Read the model definition and answer for the solid it produces. Units are mm, in the model's axes. A direction names the side the tool comes from. Give positions to 0.01 mm unless a question says otherwise; leave off trailing zeros. Loops run counter-clockwise (first coordinate to the right, second up) from the corner with the lowest first, then second, coordinate; pieces in that order, holes last. Notation, with made-up numbers: (14.5, 21.5) - (27.5, 21.5) arc R9 cw to (27.5, 26.5) - close; hole circle Ø10 at (68, 42). An arc over 180 degrees is marked (long way). Write item = value, one per line.
Autodesk Inventor part; units mm, degrees
ref_plane "YZ Plane" through (0, 0, 0) normal (1, 0, 0) x (0, 1, 0)
ref_plane "XZ Plane" through (0, 0, 0) normal (0, 1, 0) x (-1, 0, 0)
ref_plane "XY Plane" through (0, 0, 0) normal (0, 0, 1) x (1, 0, 0)
sketch "스케치1" plane through (0, 0, 0) normal (0, 0, 1) x (1, 0, 0)
  line L0 (-8.75, -14) -> (8.75, -14)
  line L1 (8.75, -14) -> (8.75, 14)
  line L2 (8.75, 14) -> (-8.75, 14)
  line L3 (-8.75, 14) -> (-8.75, -14)
  line L4 (-8.75, -14) -> (8.75, 14) construction
  line L5 (8.75, -14) -> (-8.75, 14) construction
  line L6 (-8.75, -14) -> (-6.31, -14)
  line L7 (-6.31, -14) -> (-6.31, -12.46)
  line L8 (-6.31, -12.46) -> (0, -12.46)
  line L9 (0, 0) -> (0, 2.6603)
  line L10 (8.75, -14) -> (6.31, -14)
  line L11 (6.31, -14) -> (6.31, -12.46)
  line L12 (6.31, -12.46) -> (0, -12.46)
  dimension "d0" = 17.5
  dimension "d1" = 28
  dimension "d2" = 2.44
  dimension "d3" = 1.54
extrude "돌출1" add sketch "스케치1" along normal blind 1 contours L3 L2 L1 L0 L11 L12 L8 L7
sketch "스케치2" plane through (-8.75, 14, 0) normal (0, 1, 0) x (1, 0, 0)
  line L0 (5.2, -1) -> (12.3, -1)
  line L1 (13.3, -2) -> (13.3, -3.15)
  line L2 (12.3, -4.15) -> (5.2, -4.15)
  line L3 (4.2, -3.15) -> (4.2, -2)
  line L4 (4.2, -1) -> (13.3, -4.15) construction
  line L5 (13.3, -1) -> (4.2, -4.15) construction
  line L6 (17.5, -1) -> (0, -1) construction
  line L7 (6.25, -2.075) -> (11.25, -2.075)
  line L8 (11.25, -2.075) -> (11.25, -3.075)
  line L9 (11.25, -3.075) -> (6.25, -3.075)
  line L10 (6.25, -3.075) -> (6.25, -2.075)
  line L11 (6.25, -2.075) -> (11.25, -3.075) construction
  line L12 (11.25, -2.075) -> (6.25, -3.075) construction
  arc A0 (13.3, -2) -> (12.3, -1) centre (12.3, -2) ccw
  arc A1 (12.3, -4.15) -> (13.3, -3.15) centre (12.3, -3.15) ccw
  arc A2 (5.2, -1) -> (4.2, -2) centre (5.2, -2) ccw
  arc A3 (4.2, -3.15) -> (5.2, -4.15) centre (5.2, -3.15) ccw
  line L13 (13.1, -3.15) -> (13.1, -2)
  arc A4 (13.1, -2) -> (12.3, -1.2) centre (12.3, -2) ccw
  line L14 (12.3, -1.2) -> (5.2, -1.2)
  arc A5 (5.2, -1.2) -> (4.4, -2) centre (5.2, -2) ccw
  line L15 (4.4, -2) -> (4.4, -3.15)
  arc A6 (4.4, -3.15) -> (5.2, -3.95) centre (5.2, -3.15) ccw
  line L16 (5.2, -3.95) -> (12.3, -3.95)
  arc A7 (12.3, -3.95) -> (13.1, -3.15) centre (12.3, -3.15) ccw
  point P0 (8.75, 0)
  point P1 (8.75, -2.575)
  point P2 (8.75, -1)
  dimension "d6" = 3.15
  dimension "d7" = 9.1
  dimension "d8" = 5
  dimension "d9" = 1
  dimension "d10" = 1
  dimension "d11" = 0.2
extrude "돌출2" add sketch "스케치2" along normal blind 1.74 and the other way blind 5.86
fillet "모깎기1" radius 0.7 2 edges at (6.31, -12.46, 0.5) (-6.31, -12.46, 0.5)
sketch "스케치3" plane through (-8.75, 8.14, 0) normal (0, -1, 0) x (1, 0, 0)
  line L0 (12.3, 4.15) -> (5.2, 4.15)
  arc A0 (5.2, 4.15) -> (4.2, 3.15) centre (5.2, 3.15) ccw
  line L1 (4.2, 3.15) -> (4.2, 2)
  arc A1 (4.2, 2) -> (5.2, 1) centre (5.2, 2) ccw
  line L2 (12.3, 1) -> (5.2, 1)
  arc A2 (12.3, 1) -> (13.3, 2) centre (12.3, 2) ccw
  line L3 (13.3, 2) -> (13.3, 3.15)
  arc A3 (13.3, 3.15) -> (12.3, 4.15) centre (12.3, 3.15) ccw
  arc A4 (13.1, 3.15) -> (12.3, 3.95) centre (12.3, 3.15) ccw
  line L4 (13.1, 3.15) -> (13.1, 2)
  arc A5 (12.3, 1.2) -> (13.1, 2) centre (12.3, 2) ccw
  line L5 (12.3, 1.2) -> (5.2, 1.2)
  arc A6 (4.4, 2) -> (5.2, 1.2) centre (5.2, 2) ccw
  line L6 (4.4, 2) -> (4.4, 3.15)
  arc A7 (5.2, 3.95) -> (4.4, 3.15) centre (5.2, 3.15) ccw
  line L7 (5.2, 3.95) -> (12.3, 3.95)
  point P0 (8.75, 0)
extrude "돌출3" add sketch "스케치3" against normal blind 1 contours A3 L3 A2 L2 A1 L1 A0 L0 | L4 A5 L5 A6 L6 A7 L7 A4
sketch "스케치4" plane through (0, 0, 1) normal (0, 0, 1) x (1, 0, 0)
  line L0 (3.631, 5.9375) -> (-2.5, 5.9375)
  line L1 (-2.5, 5.9375) -> (-2.5, -0.6101)
  line L2 (-2.5, -0.6101) -> (3.631, -0.6101)
  line L3 (3.631, -0.6101) -> (3.631, 5.9375)
  line L4 (3.631, 5.9375) -> (-2.5, -0.6101) construction
  line L5 (-2.5, 5.9375) -> (3.631, -0.6101) construction
  point P0 (0, 0)
  point P1 (0.5655, 2.6637)
extrude "돌출4" add sketch "스케치4" along normal blind 1.5
properties part number "C타입 충전단자"
1) A cutting plane is placed at A-A on z = 0.35. Determine the outline of the cut face in (x, y), then the cut area to 3 significant figures.
Output:
outline = (-8.75, -14) - (-6.31, -14) - (-6.31, -13.16) arc R0.7 cw to (-5.61, -12.46) - (5.61, -12.46) arc R0.7 cw to (6.31, -13.16) - (6.31, -14) - (8.75, -14) - (8.75, 14) - (-8.75, 14) - close
area = 471 mm²
2) Each of these flat-tipped pins is pushed along its axis until it touches: P1, Ø2, axis at x = 0, z = 1, coming from the -Y side; P2, Ø1.1, axis at x = -2, z = 0.5, coming from the +Y side; P3, Ø0.6, axis at y = 11, z = 2.5, coming from the -X side. Where does it stop, or does it pass through?
Output:
P1 = -12.46
P2 = 15.74
P3 = -4.55
3) A cutting plane is placed at D-D on x = 4. Determine the outline of the cut face in (y, z).
Output:
outline = (-12.46, 0) - (14, 0) - (14, 1) - (-12.46, 1) - close; (8.14, 1.11) - (15.74, 1.11) - (15.74, 1.34) - (9.14, 1.34) - (9.14, 3.81) - (15.74, 3.81) - (15.74, 4.04) - (8.14, 4.04) - close
4) A cutting plane is placed at C-C on y = -0.25. Determine the outline of the cut face in (x, z), then the cut area to 3 significant figures.
Output:
outline = (-8.75, 0) - (8.75, 0) - (8.75, 1) - (3.63, 1) - (3.63, 2.5) - (-2.5, 2.5) - (-2.5, 1) - (-8.75, 1) - close
area = 26.7 mm²
5) The mould has two halves that part along X. Classify faces 5 (the face through (-4.11, 12.39, 3.72)), 6 (the face through (8.75, -0.2, 0.5)), 7 (the face through (-4.249, 11.887, 3.865)): pulls with the +X half, pulls with the -X half, needs draft (parallel to the pull), parting line crosses it, or undercut.
Output:
face_5 = undercut
face_6 = pulls with the +X half
face_7 = pulls with the -X half
6) A tool of negligible diameter and unlimited length cuts with its end or side. For faces 1 (the face through (1, -0.61, 2)), 2 (the face through (3.631, 3, 2)), 3 (the face through (0, 12, 3.075)), 4 (the face through (6.31, -13.6, 0.5)), from which of +Z, -Z, +X, -X, +Y, -Y can it reach the whole face along a straight path? Write none if from no direction.
Output:
face_1 = +Z, +X, -X, -Y
face_2 = +Z, +X, -Y
face_3 = +Y
face_4 = +Z, -Z, -Y
7) Find the intervals of material crossed by probe 1 along X at (y, z) = (12.25, 2.3); probe 2 along Z at (x, y) = (2, 11.75) (3 decimals); probe 3 along Z at (x, y) = (-7, -0.25), in increasing order.
Output:
probe_1 = -4.55 to -4.35, -2.5 to 2.5, 4.35 to 4.55
probe_2 = 0 to 1.2, 2.075 to 3.075, 3.95 to 4.15
probe_3 = 0 to 1
